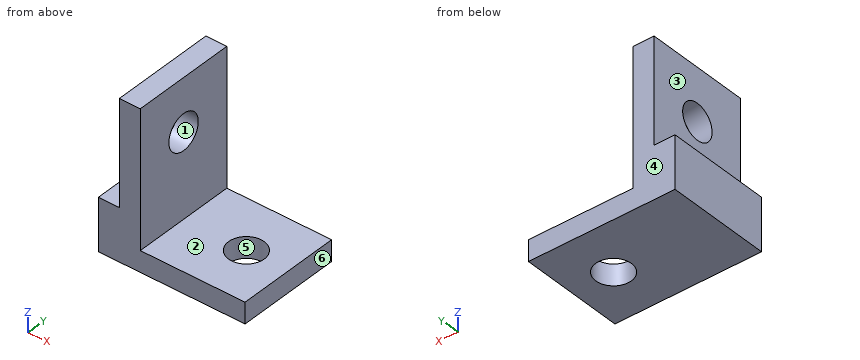
```python
from build123d import *

# Parameters (mm, degrees)
F1_DEPTH = 10
F3_D     = 3.4
F5_D     = 3.4


with BuildPart() as f1:
    # F0 (on Front) → F1 (new body)
    with BuildSketch(Plane.XZ):
        Polygon((0, 5), (0, 0), (14, 0), (14, 2), (4, 2), (4, 15), (2, 15), (2, 5), align=None)
    extrude(amount=F1_DEPTH)

    # F3 (through all)
    with Locations(Plane.YZ.offset(4)):
        with Locations((-5, 10)):
            Hole(F3_D / 2)

    # F5 (through all)
    with Locations(Plane.XY.offset(2)):
        with Locations((10, -5)):
            Hole(F5_D / 2)


solid = f1.part
```
Geometry: final body of the model. Coordinates: model frame, mm. Face numbers are marked on the shaded views. A direction names the side the tool comes from. Coordinates: 2 decimals unless noted, no trailing zeros. Loops run counter-clockwise (first coordinate to the right, second up) from the corner with the lowest first, then second, coordinate; pieces in that order, holes last. Notation, with made-up numbers: (81, -30) -> (109, -30) arc R22 ccw to (109, 3) -> close; hole circle Ø9 at (-6.75, -23). An arc over 180 degrees is marked (long way). Use a Markdown table: item, result. Add a question column.
(1) Line query: line 1 along X through (y, z) = (-5.75, 2.25); line 2 along Y through (x, z) = (10, 0.95); line 3 along X through (y, z) = (-8.25, 13.25). Output: solid intervals per line, ascending.
(2) Access query for the marked faces 1, 2 and 3. Directions: +Z, -Z, +X, -X, +Y, -Y. A direction counts if a zero-diameter tool reaches every point of the face in a straight line with its end or side. Return the directions, or none.
(3) Section query C-C, the plane z = 10. Return loops of the section in (x, y).
(4) Section query D-D, the plane y = -8.25. Return loops of the section in (x, z).
(5) Section query B-B, the plane y = -5. Return loops of the section in (x, z), plus the area to 3 significant figures.
(6) Pin query (flat end, axial travel): pin 1 Ø2 at (y, z) = (-5, 10) entering from -X; pin 2 Ø1 at (x, y) = (10.5, -2) entering from +Z; pin 3 Ø5 at (y, z) = (-5, 12.5) entering from +X. Return the tip coordinate at first contact, or that it passes through.
(7) Section query A-A, the plane x = 10. Return loops of the section in (y, z), plus the area to 3 significant figures.
(8) Mould query, pull axis Y, two halves, no side actions, for the marked faces 4, 5 and 6. Classes: pulls with the +Y half, pulls with the -Y half, needs draft (parallel to the pull), parting line crosses it, or undercut.
Answer:
| question | item | result |
|---|---|---|
| 1 | line 1 | x = 0 to 4 |
| 1 | line 2 | y = -10 to -6.7, -3.3 to 0 |
| 1 | line 3 | x = 2 to 4 |
| 2 | face 1 | +X, -X |
| 2 | face 2 | +Z, +X, +Y, -Y |
| 2 | face 3 | +Z, -X, +Y, -Y |
| 3 | outline | (2, -10) -> (4, -10) -> (4, -6.7) -> (2, -6.7) -> close; (2, -3.3) -> (4, -3.3) -> (4, 0) -> (2, 0) -> close |
| 4 | outline | (0, 0) -> (14, 0) -> (14, 2) -> (4, 2) -> (4, 15) -> (2, 15) -> (2, 5) -> (0, 5) -> close |
| 5 | outline | (0, 0) -> (8.3, 0) -> (8.3, 2) -> (4, 2) -> (4, 8.3) -> (2, 8.3) -> (2, 5) -> (0, 5) -> close; (2, 11.7) -> (4, 11.7) -> (4, 15) -> (2, 15) -> close; (11.7, 0) -> (14, 0) -> (14, 2) -> (11.7, 2) -> close |
| 5 | area | 46.4 mm^2 |
| 6 | pin 1 | passes through |
| 6 | pin 2 | stops at z = 2 |
| 6 | pin 3 | stops at x = 4 |
| 7 | outline | (-10, 0) -> (-6.7, 0) -> (-6.7, 2) -> (-10, 2) -> close; (-3.3, 0) -> (0, 0) -> (0, 2) -> (-3.3, 2) -> close |
| 7 | area | 13.2 mm^2 |
| 8 | face 4 | pulls with the +Y half |
| 8 | face 5 | undercut |
| 8 | face 6 | needs draft |
